Verification items for the finished model (mm, model axes). Face numbers are marked on the shaded views. A direction names the side the tool comes from. Coordinates: 2 decimals unless noted, no trailing zeros. Write each loop counter-clockwise with the first axis right and the second up, starting at its lowest first coordinate (ties: lowest second). Pieces come first, ordered by that corner, then holes. Notation, with made-up numbers: (41.25, 84) -> (69.25, 84) arc R10 cw to (69.25, 99) -> close; hole circle Ø11 at (68, 28.25). An arc over 180 degrees is marked (long way). Answer in a Markdown table with one row per item.
```python
from build123d import *

# Parameters (mm, degrees)
SKETCH1_R           = 7.5
BOSS_EXTRUDE1_DEPTH = 2
SKETCH2_R           = 3
BOSS_EXTRUDE2_DEPTH = 2
SKETCH3_R           = 0.655
CUT_EXTRUDE1_DEPTH  = 2.89
SKETCH4_R           = 0.655
CUT_EXTRUDE3_DEPTH  = 1.11
CUT_EXTRUDE3_DRAFT  = 60


with BuildPart() as part:
    # Sketch1 → Boss-Extrude1 (new body)
    with BuildSketch(Plane(origin=(0, 0, 0), x_dir=(1, 0, 0), z_dir=(0, 1, 0))):
        with Locations(Location((0, 0, 0), (0, 0, 270))):
            Circle(SKETCH1_R)
    extrude(amount=BOSS_EXTRUDE1_DEPTH)

    # Sketch2 → Boss-Extrude2 (add)
    with BuildSketch(Plane(origin=(0, 2, 0), x_dir=(1, 0, 0), z_dir=(0, 1, 0))):
        with Locations(Location((0, 0, 0), (0, 0, 270))):
            Circle(SKETCH2_R)
    extrude(amount=BOSS_EXTRUDE2_DEPTH)

    # Sketch3 → Cut-Extrude1 (cut)
    with BuildSketch(Plane(origin=(0, 4, 0), x_dir=(1, 0, 0), z_dir=(0, 1, 0))):
        with Locations(Location((0, 0, 0), (0, 0, 270))):
            Circle(SKETCH3_R)
    extrude(amount=-CUT_EXTRUDE1_DEPTH, mode=Mode.SUBTRACT)


with BuildPart() as cut_extrude3_tool:
    # Sketch4 → Cut-Extrude3 (with draft: the straight prism first)
    with BuildSketch(Plane(origin=(0, 1.11, 0), x_dir=(1, 0, 0), z_dir=(0, 1, 0))):
        with Locations(Location((0, 0, 0), (0, 0, 270))):
            Circle(SKETCH4_R)
    extrude(amount=-CUT_EXTRUDE3_DEPTH)
    # Cut-Extrude3: the draft: its side faces are tilted about the plane it starts from
    cut_extrude3_sides = [cut_extrude3_tool.faces().sort_by_distance(p)[0] for p in [
        (0, 0.555, -0.655),
    ]]
    draft(cut_extrude3_sides, Plane(origin=(0, 1.11, 0), x_dir=(1, 0, 0), z_dir=(0, 1, 0)), CUT_EXTRUDE3_DRAFT)


with BuildPart() as part_1:
    add(part.part)

    # Cut-Extrude3: cut by cut_extrude3_tool
    add(cut_extrude3_tool.part, mode=Mode.SUBTRACT)


solid = part_1.part
```
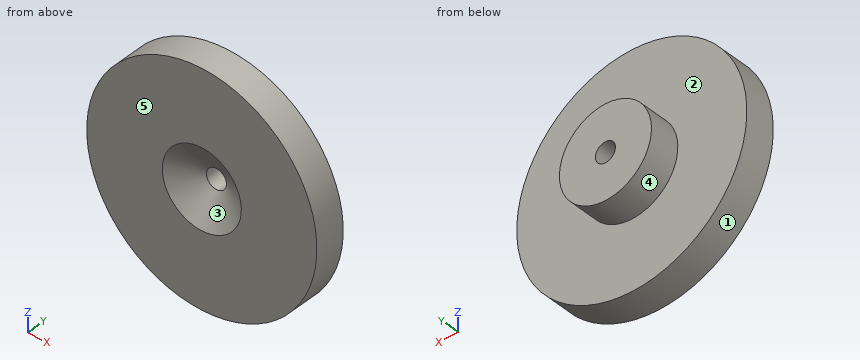
1. Sectioned sample at B-B, the plane x = 0. Record the cut outline in (y, z) (3 decimals).
Findings below:
| item | result |
|---|---|
| outline | (0, -7.5) -> (2, -7.5) -> (2, -3) -> (4, -3) -> (4, -0.655) -> (1.11, -0.655) -> (0, -2.578) -> close; (0, 2.578) -> (1.11, 0.655) -> (4, 0.655) -> (4, 3) -> (2, 3) -> (2, 7.5) -> (0, 7.5) -> close |
2. Go/stop test with flat-tipped pins: pin 1 (1.5 mm diameter, centred on x = -1, y = 1, fed in from -Z); pin 2 (1 mm diameter, centred on y = 3, z = 4.5, fed in from +X); pin 3 (1.5 mm diameter, centred on y = 1, z = -0.5, fed in from +X); pin 4 (1.5 mm diameter, centred on x = -4.5, y = 1.5, fed in from +Z). Record where each tip stops, or that it passes through.
Findings below:
| item | result |
|---|---|
| pin 1 | stops at z = -7.5 |
| pin 2 | passes through |
| pin 3 | stops at x = 7.5 |
| pin 4 | stops at z = 6.5 |
3. Sectioned sample at D-D, the plane z = 6.5. Record the cut outline in (x, y), and give its area (3 significant figures).
Findings below:
| item | result |
|---|---|
| outline | (-3.74, 0) -> (3.74, 0) -> (3.74, 2) -> (-3.74, 2) -> close |
| area | 15.0 mm² |
4. Sectioned sample at C-C, the plane y = 1.35. Record the cut outline in (x, z) (3 decimals), and give its area (3 significant figures).
Findings below:
| item | result |
|---|---|
| outline | circle Ø15 at (0, 0); hole circle Ø1.31 at (0, 0) |
| area | 175 mm² |
5. Release check for a two-part mould opening along X. For the marked faces 1, 2 and 3 record: released by +X, released by -X, zero draft, split by the parting line, or undercut.
Findings below:
| item | result |
|---|---|
| face 1 | split by the parting line |
| face 2 | zero draft |
| face 3 | undercut |
6. Sectioned sample at A-A, the plane z = 0. Record the cut outline in (x, y) (3 decimals).
Findings below:
| item | result |
|---|---|
| outline | (-7.5, 0) -> (-2.578, 0) -> (-0.655, 1.11) -> (-0.655, 4) -> (-3, 4) -> (-3, 2) -> (-7.5, 2) -> close; (0.655, 1.11) -> (2.578, 0) -> (7.5, 0) -> (7.5, 2) -> (3, 2) -> (3, 4) -> (0.655, 4) -> close |
7. Access from +Z, -Z, +X, -X, +Y, -Y to the whole of each face (thin tool, end or side, straight path). Record for the marked faces 4 and 5.
Findings below:
| item | result |
|---|---|
| face 4 | +Y |
| face 5 | +Z, -Z, +X, -X, -Y |
8. Material ranges on probe 1 along X at (y, z) = (3, 0) (3 decimals); probe 2 along Y at (x, z) = (3.75, 4.75); probe 3 along X at (y, z) = (1.45, -0.5), recorded low to high. Write a range as from..to.
Findings below:
| item | result |
|---|---|
| probe 1 | x = -3..-0.655, 0.655..3 |
| probe 2 | y = 0..2 |
| probe 3 | x = -7.48..-0.42, 0.42..7.48 |
